Answer from the drawing. Dimensions are ordinates in mm from the lowest x, y and z of the part. A direction names the side the tool comes from. Round coordinates to 2 decimals unless told otherwise and drop trailing zeros. Loops run counter-clockwise (first coordinate to the right, second up) from the corner with the lowest first, then second, coordinate; pieces in that order, holes last. Notation, with made-up numbers: M 50.5,-13 L 68.5,-13 A31 ccw 68.5,15 Z; hole C 13.25,-9 d2. An arc over 180 degrees is marked long. One line per item, written item: value.
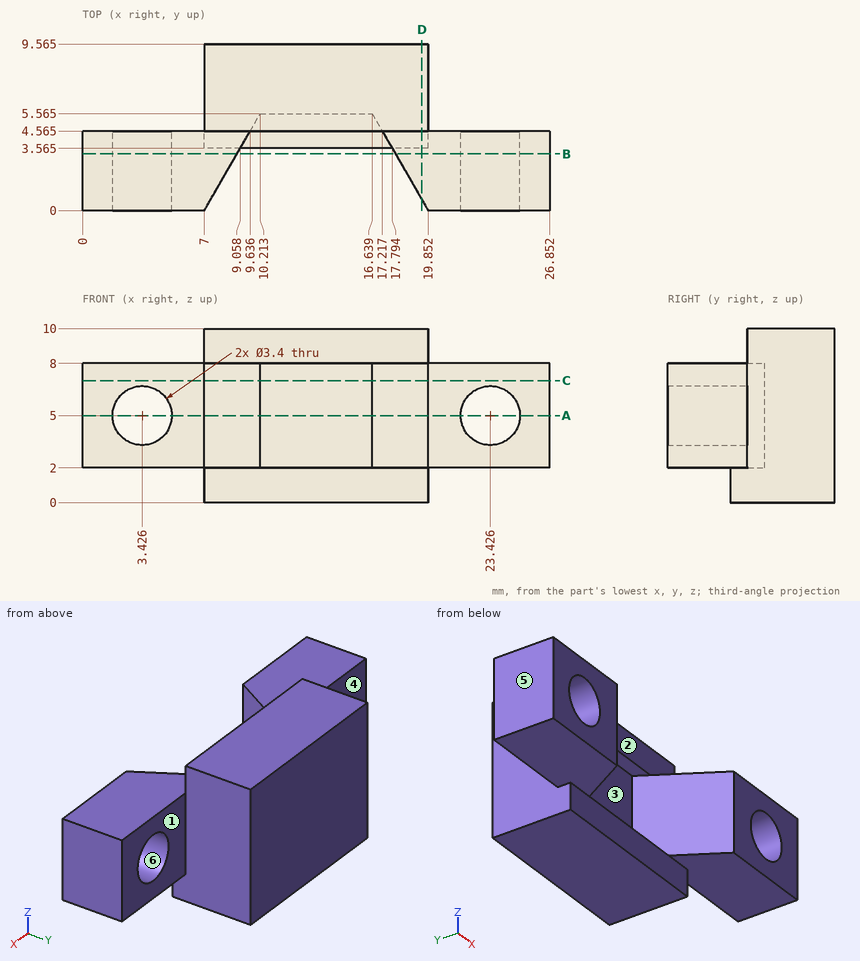
1) The mould has two halves that part along X. Classify the marked faces 4, 5 and 6: +X half, -X half, draft (parallel to the pull), parting line (faces both ways), or undercut.
Check values:
face 4: draft
face 5: -X half
face 6: undercut
2) Find the intervals of material crossed by probe 1 along Z at (x, y) = (3.5, 4.25); probe 2 along X at (y, z) = (1.2, 5) (1 decimal); probe 3 along Y at (x, z) = (10.5, 4.25) (1 decimal), in increasing order. Write a range as from..to.
Check values:
probe 1: 2..3.3, 6.7..8
probe 2: 0..1.7, 5.1..7.7, 19.2..21.7, 25.1..26.9
probe 3: 5.6..9.6
3) Find section A-A (z = 5). Give the vertices of the cut face in (x, y) (1 decimal).
Check values:
outline: M 0,0 L 1.7,0 L 1.7,4.6 L 0,4.6 Z; M 5.1,0 L 7,0 L 10.2,5.6 L 16.6,5.6 L 19.9,0 L 21.7,0 L 21.7,4.6 L 19.9,4.6 L 19.9,9.6 L 7,9.6 L 7,4.6 L 5.1,4.6 Z; M 25.1,0 L 26.9,0 L 26.9,4.6 L 25.1,4.6 Z
4) For the marked faces 1, 2 and 3, determine the directions among +Z, -Z, +X, -X, +Y, -Y from which every point of the face is accessible in a straight line to the end or side of a thin tool.
Check values:
face 1: +Z, -Z, +X, +Y
face 2: +Z, +X, -X, -Y
face 3: -Y
5) Find section D-D (x = 19.5). Give the vertices of the cut face in (y, z) (1 decimal).
Check values:
outline: M 0.6,2 L 3.6,2 L 3.6,0 L 9.6,0 L 9.6,10 L 4.6,10 L 4.6,8 L 0.6,8 Z
6) Find section C-C (z = 7). Give the vertices of the cut face in (x, y) (1 decimal).
Check values:
outline: M 0,0 L 7,0 L 10.2,5.6 L 16.6,5.6 L 19.9,0 L 26.9,0 L 26.9,4.6 L 19.9,4.6 L 19.9,9.6 L 7,9.6 L 7,4.6 L 0,4.6 Z
7) Find section B-B (y = 3.25). Give the vertices of the cut face in (x, z).
Check values:
outline: M 0,2 L 8.88,2 L 8.88,8 L 0,8 Z; M 17.98,2 L 26.85,2 L 26.85,8 L 17.98,8 Z; hole C 3.43,5 d3.4; hole C 23.43,5 d3.4
8) Each of these flat-tipped pins is pushed along its axis until it touches: pin 1 (5 mm diameter, centred on x = 12.5, z = 4, fed in from -Y) (1 decimal); pin 2 (1.4 mm diameter, centred on x = 22.5, y = 1.5, fed in from -Z); pin 3 (5 mm diameter, centred on y = 8, z = 1.5, fed in from -X). Where does it stop, or does it pass through?
Check values:
pin 1: y = 3.6
pin 2: z = 2
pin 3: x = 7
